Autodesk Inventor part; units mm, degrees
ref_plane "YZ Plane" through (0, 0, 0) normal (1, 0, 0) x (0, 1, 0)
ref_plane "XZ Plane" through (0, 0, 0) normal (0, 1, 0) x (-1, 0, 0)
ref_plane "XY Plane" through (0, 0, 0) normal (0, 0, 1) x (1, 0, 0)
sketch "Sketch1" plane through (0, 0, 0) normal (0, 0, 1) x (1, 0, 0)
  line L0 (0, 0) -> (22, 0)
  line L1 (22, 0) -> (22, 10)
  line L2 (22, 10) -> (0, 10)
  line L3 (0, 10) -> (0, 0)
  circle A0 centre (17, 5) radius 1.5
  circle A1 centre (2, 5) radius 1
  point P0 (22, 5)
  dimension "d0" = 22
  dimension "d1" = 10
  dimension "d2" = 3
  dimension "d3" = 2
  dimension "d4" = 15
  dimension "d5" = 5
extrude "Extrusion1" add sketch "Sketch1" along normal blind 2
fillet "Fillet1" radius 4 2 edges at (22, 10, 1) (22, 0, 1)
chamfer "Chamfer1" distance 3 angle 45 2 edges at (0, 10, 1) (0, 0, 1)
properties part number "servo arm"
Here's how the part is built. I have some questions about the finished solid (model axes, mm). Round coordinates to 2 decimals unless told otherwise and drop trailing zeros. Order: outer loops, then holes, each group sorted by start corner. A loop starts at its lowest first (then second) coordinate and runs counter-clockwise, first axis right, second up. Notation, with made-up numbers: M -19,-25.75 L -14,-25.75 A18 cw -14,-8.75 Z; hole C 64.5,28 d7. An arc over 180 degrees is marked long. Return JSON: item names as keys, results as strings. Group by question number.
1. If we section it at D-D on x = 2: List the corners of the cut face in (y, z) for me, then the cut area to 3 significant figures.
2. If we section it at C-C on z = 1.2: List the corners of the cut face in (x, y) for me.
3. If we section it at A-A on y = 5: List the corners of the cut face in (x, z) for me, then the cut area to 3 significant figures.
4. Please list where these lines run through material, in increasing order: probe 1 along X at (y, z) = (4.5, 1.95); probe 2 along Y at (x, z) = (17, 0.85); probe 3 along Y at (x, z) = (15.75, 0.5).
5. If we section it at B-B on x = 17: List the corners of the cut face in (y, z) for me, then the cut area to 3 significant figures.
Reply:
{
 "1": {"outline": "M 1,0 L 4,0 L 4,2 L 1,2 Z; M 6,0 L 9,0 L 9,2 L 6,2 Z", "area": "12.0 mm^2"},
 "2": {"outline": "M 0,3 L 3,0 L 18,0 A4 ccw 22,4 L 22,6 A4 ccw 18,10 L 3,10 L 0,7 Z; hole C 2,5 d2; hole C 17,5 d3"},
 "3": {"outline": "M 0,0 L 1,0 L 1,2 L 0,2 Z; M 3,0 L 15.5,0 L 15.5,2 L 3,2 Z; M 18.5,0 L 22,0 L 22,2 L 18.5,2 Z", "area": "34.0 mm^2"},
 "4": {"probe 1": "0 to 1.13, 2.87 to 15.59, 18.41 to 22", "probe 2": "0 to 3.5, 6.5 to 10", "probe 3": "0 to 4.17, 5.83 to 10"},
 "5": {"outline": "M 0,0 L 3.5,0 L 3.5,2 L 0,2 Z; M 6.5,0 L 10,0 L 10,2 L 6.5,2 Z", "area": "14.0 mm^2"}
}
